```python
from build123d import *

# Parameters (mm, degrees)
SKETCH1_R           = 25.5
BOSS_EXTRUDE1_DEPTH = 116
SKETCH3_OUTSIDE_W   = 80.318
SKETCH3_OUTSIDE_H   = 80.318
SKETCH3_OUTSIDE_R   = 11
CUT_EXTRUDE2_DEPTH  = 18
SKETCH4_W           = 35.319317214
SKETCH4_H           = 8
CUT_EXTRUDE3_DEPTH  = 12
SKETCH5_W           = 64
SKETCH5_H           = 71.607933851
SKETCH5_R           = 2.910259783
SKETCH5_R_2         = 2.987781855
SKETCH5_R_3         = 2.610532629
SKETCH5_R_4         = 2.006978968
BOSS_EXTRUDE2_DEPTH = 8
SKETCH6_R           = 10
BOSS_EXTRUDE3_DEPTH = 20


with BuildPart() as part:
    # Sketch1 → Boss-Extrude1 (new body)
    with BuildSketch(Plane.XY):
        with Locations(Location((0, 0, 0), (0, 0, 180))):
            Circle(SKETCH1_R)
    extrude(amount=BOSS_EXTRUDE1_DEPTH)

    # Sketch3 outside → Cut-Extrude2 (cut)
    with BuildSketch(Plane(origin=(0, 0, 0), x_dir=(-1, 0, 0), z_dir=(0, 0, -1))):
        Rectangle(SKETCH3_OUTSIDE_W, SKETCH3_OUTSIDE_H)
        Circle(SKETCH3_OUTSIDE_R, mode=Mode.SUBTRACT)
    extrude(amount=-CUT_EXTRUDE2_DEPTH, mode=Mode.SUBTRACT)

    # Sketch4 → Cut-Extrude3 (cut)
    with BuildSketch(Plane(origin=(0, 0, 0), x_dir=(-1, 0, 0), z_dir=(0, 0, -1))):
        with Locations((-2.725981742, 0)):
            Rectangle(SKETCH4_W, SKETCH4_H)
    extrude(amount=-CUT_EXTRUDE3_DEPTH, mode=Mode.SUBTRACT)

    # Sketch5 → Boss-Extrude2 (add)
    with BuildSketch(Plane(origin=(0, 32, 0), x_dir=(-1, 0, 0), z_dir=(0, 1, 0))):
        with Locations((0, 68.315264107)):
            Rectangle(SKETCH5_W, SKETCH5_H)
        with Locations(Location((-25, 90, 0), (0, 0, 90))):
            Circle(SKETCH5_R, mode=Mode.SUBTRACT)
        with Locations(Location((-25, 40, 0), (0, 0, 90))):
            Circle(SKETCH5_R_2, mode=Mode.SUBTRACT)
        with Locations(Location((25, 90, 0), (0, 0, 90))):
            Circle(SKETCH5_R_3, mode=Mode.SUBTRACT)
        with Locations(Location((25, 40, 0), (0, 0, 90))):
            Circle(SKETCH5_R_4, mode=Mode.SUBTRACT)
    extrude(amount=-BOSS_EXTRUDE2_DEPTH)

    # Sketch6 → Boss-Extrude3 (add)
    with BuildSketch(Plane.XY.offset(116)):
        Circle(SKETCH6_R)
    extrude(amount=BOSS_EXTRUDE3_DEPTH)


solid = part.part
```
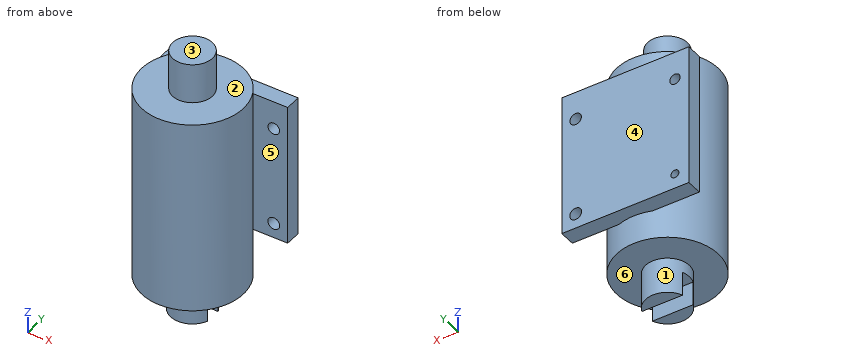
Design review of the part built by this model. Coordinates are the model's own, in mm. Face numbers are marked on the shaded views. A direction names the side the tool comes from. Give positions to 0.01 mm unless a question says otherwise; leave off trailing zeros. Loops run counter-clockwise (first coordinate to the right, second up) from the corner with the lowest first, then second, coordinate; pieces in that order, holes last. Notation, with made-up numbers: M -33.75,33.25 L 19.25,33.25 A29 ccw 19.25,68.25 Z; hole C -10.5,43 d7. An arc over 180 degrees is marked long. Return JSON: item names as keys, results as strings. Group by question number.
Item 1: We need section C-C (x = -19). Give the boundary of the cut face in (y, z), and give its area (3 significant figures).
Item 2: We need section B-B (y = 0). Give the boundary of the cut face in (x, z).
Item 3: We need section A-A (z = 90). Give the boundary of the cut face in (x, y).
Item 4: Insertion check: pin 1 Ø2 at (x, z) = (18.5, 67.5) entering from -Y; pin 2 Ø13 at (x, z) = (1, 6) entering from -Y; pin 3 Ø5 at (x, z) = (25, 90) entering from -Y. Each pin has a flat end and moves straight along its axis. Give the tip position at first contact, or say it passes through.
Item 5: We need section D-D (x = 0). Give the boundary of the cut face in (y, z).
Item 6: Tool access review of the marked faces 1, 2 and 3: name each direction out of +Z, -Z, +X, -X, +Y, -Y from which nothing blocks a thin tool from reaching the whole face with its end or side.
Item 7: For probe 1 along X at (y, z) = (28.5, 40); probe 2 along X at (y, z) = (26, 90); probe 3 along Z at (x, y) = (-17, -7.5), list the stretches that pass through material, from the lowest coordinate up.
Item 8: Mouldability with a two-part tool opening along Y and no side actions: class the marked faces 4, 5 and 6 as released by +Y, released by -Y, zero draft, split by the parting line, or undercut.
Output:
{
 "1": {"outline": "M -17.01,18 L 17.01,18 L 17.01,116 L -17.01,116 Z; M 24,32.51 L 32,32.51 L 32,104.12 L 24,104.12 Z", "area": "3,910 mm^2"},
 "2": {"outline": "M -25.5,18 L -11,18 L -11,12 L 11,12 L 11,18 L 25.5,18 L 25.5,116 L 10,116 L 10,136 L -10,136 L -10,116 L -25.5,116 Z"},
 "3": {"outline": "M -32,24 L -27.61,24 L -27.61,32 L -32,32 Z; M -22.39,24 L -8.62,24 A25.5 ccw long 8.62,24 L 22.09,24 L 22.09,32 L -22.39,32 Z; M 27.91,24 L 32,24 L 32,32 L 27.91,32 Z"},
 "4": {"pin 1": "stops at y = -18.55", "pin 2": "stops at y = -11", "pin 3": "stops at y = -12"},
 "5": {"outline": "M -25.5,18 L -11,18 L -11,0 L -4,0 L -4,12 L 4,12 L 4,0 L 11,0 L 11,18 L 25.5,18 L 25.5,32.51 L 32,32.51 L 32,104.12 L 25.5,104.12 L 25.5,116 L 10,116 L 10,136 L -10,136 L -10,116 L -25.5,116 Z"},
 "6": {"face 1": "-Z", "face 2": "+Z", "face 3": "+Z, +X, -X, +Y, -Y"},
 "7": {"probe 1": "x = -32 to -27.01, -22.99 to 22.01, 27.99 to 32", "probe 2": "x = -32 to -27.61, -22.39 to 22.09, 27.91 to 32", "probe 3": "z = 18 to 116"},
 "8": {"face 4": "released by +Y", "face 5": "undercut", "face 6": "zero draft"}
}
